Autodesk Inventor part; units mm, degrees
ref_plane "YZ Plane" through (0, 0, 0) normal (1, 0, 0) x (0, 1, 0)
ref_plane "XZ Plane" through (0, 0, 0) normal (0, 1, 0) x (-1, 0, 0)
ref_plane "XY Plane" through (0, 0, 0) normal (0, 0, 1) x (1, 0, 0)
sketch "Sketch1" plane through (0, 0, 0) normal (0, 1, 0) x (-1, 0, 0)
  line L0 (10, 3.75) -> (-10, 3.75)
  line L1 (-10, 3.75) -> (-10, -3.75)
  line L2 (-10, -3.75) -> (10, -3.75)
  line L3 (10, -3.75) -> (10, 3.75)
  line L4 (10, 3.75) -> (-10, -3.75) construction
  line L5 (-10, 3.75) -> (10, -3.75) construction
  circle A0 centre (5, 0) radius 1.7
  circle A1 centre (-5, 0) radius 1.7
  point P0 (0, 0)
  dimension "d0" = 20
  dimension "d1" = 7.5
  dimension "d2" = 3.4
  dimension "d3" = 3.4
  dimension "d4" = 5
  dimension "d5" = 5
extrude "Extrusion1" add sketch "Sketch1" along normal blind 30
fillet "Fillet1" radius 3 4 edges at (10, 15, 3.75) (10, 15, -3.75) (-10, 15, -3.75) (-10, 15, 3.75)
properties part number "b1"
Source: CAD feature listing. Evaluate the final solid. Frame: model axes, mm. Round coordinates to 2 decimals unless told otherwise and drop trailing zeros. Loops run counter-clockwise (first coordinate to the right, second up) from the corner with the lowest first, then second, coordinate; pieces in that order, holes last.
1. Section query C-C on y = 10.75. Output: boundary loops of the cut face in (x, z), and give its area (3 significant figures).
2. Section query B-B on x = -5. Output: boundary loops of the cut face in (y, z).
3. Section query D-D on x = 5.5. Output: boundary loops of the cut face in (y, z), and give its area (3 significant figures).
4. Ray query, L1, parallel to Z at x = -5, y = 12; L2, parallel to X at y = 20, z = 1.5; L3, parallel to Z at x = 5.5, y = 8. Return the intervals inside material, ascending.
5. Section query A-A on z = 0. Output: boundary loops of the cut face in (x, y).
6. Mould query, pull axis X, two halves, no side actions, for faces 1 (the flat face through (0, 0, 0)), 2 (the cylindrical face through (3.43, 14.79, 0.65)), 3 (the cylindrical face through (-9.1, 15.21, -2.89)). Classes: released by +X, released by -X, zero draft, split by the parting line, or undercut.
Answers below:
1. outline: (-10, -0.75) arc R3 ccw to (-7, -3.75) - (7, -3.75) arc R3 ccw to (10, -0.75) - (10, 0.75) arc R3 ccw to (7, 3.75) - (-7, 3.75) arc R3 ccw to (-10, 0.75) - close; hole circle Ø3.4 at (-5, 0); hole circle Ø3.4 at (5, 0)
1. area: 124 mm2
2. outline: (0, -3.75) - (30, -3.75) - (30, -1.7) - (0, -1.7) - close; (0, 1.7) - (30, 1.7) - (30, 3.75) - (0, 3.75) - close
3. outline: (0, -3.75) - (30, -3.75) - (30, -1.62) - (0, -1.62) - close; (0, 1.62) - (30, 1.62) - (30, 3.75) - (0, 3.75) - close
3. area: 128 mm2
4. L1: z = -3.75 to -1.7, 1.7 to 3.75
4. L2: x = -9.9 to -5.8, -4.2 to 4.2, 5.8 to 9.9
4. L3: z = -3.75 to -1.62, 1.62 to 3.75
5. outline: (-10, 0) - (-6.7, 0) - (-6.7, 30) - (-10, 30) - close; (-3.3, 0) - (3.3, 0) - (3.3, 30) - (-3.3, 30) - close; (6.7, 0) - (10, 0) - (10, 30) - (6.7, 30) - close
6. face 1: zero draft
6. face 2: undercut
6. face 3: released by -X
